from build123d import *

# Parameters (mm, degrees)
SKETCH_1_R               = 4
EXTRUDE_1_DEPTH          = 74.5
CUT_EXTRUDE_1_DEPTH      = 75.714456432
CUT_EXTRUDE_1_DEPTH_BACK = 75.714456432
SKETCH_2_W               = 2
SKETCH_2_H               = 6


with BuildPart() as part:
    # 草图1 → 凸台-拉伸1 (new, symmetric)
    with BuildSketch(Plane.XY):
        Circle(SKETCH_1_R)
    extrude(amount=EXTRUDE_1_DEPTH, both=True)

    # 草图2 → 切除-拉伸1 (cut, two sides: drawn at the far end of the back side and taken through both)
    with BuildSketch(Plane(origin=(0, 0, 0), x_dir=(1, 0, 0), z_dir=(0, 1, 0)).offset(-CUT_EXTRUDE_1_DEPTH_BACK)):
        with Locations((-3, -71.5)):
            Rectangle(SKETCH_2_W, SKETCH_2_H)
        with Locations((3, -71.5)):
            Rectangle(SKETCH_2_W, SKETCH_2_H)
    extrude(amount=CUT_EXTRUDE_1_DEPTH + CUT_EXTRUDE_1_DEPTH_BACK, mode=Mode.SUBTRACT)


solid = part.part
Work out the finished part from the listing and answer in its coordinate system (mm). A direction names the side the tool comes from. Give positions to 0.01 mm unless a question says otherwise; leave off trailing zeros. Loops run counter-clockwise (first coordinate to the right, second up) from the corner with the lowest first, then second, coordinate; pieces in that order, holes last. Notation, with made-up numbers: (58.5, 30.5) - (68.5, 30.5) arc R16 cw to (68.5, 51.5) - close; hole circle Ø3 at (27.25, 21.5). An arc over 180 degrees is marked (long way). Answer in a Markdown table with one row per item.
(1) Flat-ended cylindrical pins translate along their axes: pin 1 Ø3 at (y, z) = (-1, 71.5) entering from +X; pin 2 Ø3 at (y, z) = (1, 72) entering from -X; pin 3 Ø1.6 at (x, y) = (-3.5, 1) entering from +Z. Find the tip coordinate at first contact, or state that the pin passes through.
Results list:
| item | result |
|---|---|
| pin 1 | stops at x = 2 |
| pin 2 | stops at x = -2 |
| pin 3 | stops at z = 68.5 |
(2) A tool of negligible diameter and unlimited length cuts with its end or side. For faces 1 (the face through (-2, 0, 72)), 2 (the face through (2, 0, 72)), 3 (the face through (0, 0, 74.5)), from which of +Z, -Z, +X, -X, +Y, -Y can it reach the whole face along a straight path? Write none if from no direction.
Results list:
| item | result |
|---|---|
| face 1 | +Z, -X, +Y, -Y |
| face 2 | +Z, +X, +Y, -Y |
| face 3 | +Z, +X, -X, +Y, -Y |
(3) Consider L1, parallel to X at y = 2, z = -52; L2, parallel to Z at x = 2.5, y = -2.75. Determine where each line is inside the solid, lowest interval first. Write a range as [from, to].
Results list:
| item | result |
|---|---|
| L1 | x = [-3.46, 3.46] |
| L2 | z = [-74.5, 68.5] |
(4) Section A-A (y = 0) is taken. Give the vertices of the cut face in (x, z), and give its area (3 significant figures).
Results list:
| item | result |
|---|---|
| outline | (-4, -74.5) - (4, -74.5) - (4, 68.5) - (2, 68.5) - (2, 74.5) - (-2, 74.5) - (-2, 68.5) - (-4, 68.5) - close |
| area | 1,170 mm² |
(5) Section B-B (z = 50) is taken. Give the vertices of the cut face in (x, y), and give its area (3 significant figures).
Results list:
| item | result |
|---|---|
| outline | circle Ø8 at (0, 0) |
| area | 50.3 mm² |
